Geometry: final body of the model. Coordinates: model frame, mm. Give positions to 0.01 mm unless a question says otherwise; leave off trailing zeros. Write each loop counter-clockwise with the first axis right and the second up, starting at its lowest first coordinate (ties: lowest second). Pieces come first, ordered by that corner, then holes. Notation, with made-up numbers: (-26, 79) -> (14, 79) arc R29 ccw to (14, 107) -> close; hole circle Ø6 at (-18.5, 13). An arc over 180 degrees is marked (long way). Answer in a Markdown table with one row per item. Add a question column.
Item 1: Section query B-B on x = -1.13. Output: boundary loops of the cut face in (y, z), plus the area to 3 significant figures.
Item 2: Section query D-D on y = 0.55. Output: boundary loops of the cut face in (x, z), plus the area to 3 significant figures.
Item 3: Section query A-A on z = -2. Output: boundary loops of the cut face in (x, y), plus the area to 3 significant figures.
Item 4: Material intervals for probe 1 along Z at (x, y) = (-0.65, 0.25); probe 2 along Y at (x, z) = (-1.45, 3.5); probe 3 along X at (y, z) = (-1.2, 3), sorted ascending. Write a range as from..to.
Item 5: First-contact query: P1, Ø2, axis at x = 1, z = 6.5, coming from the -Y side; P2, Ø2, axis at x = 1.5, z = -0.5, coming from the -Y side. Flat tips, straight axial feed; report the tip coordinate or a pass-through.
Item 6: Section query C-C on z = 2.5. Output: boundary loops of the cut face in (x, y).
```python
from build123d import *

# Parameters (mm, degrees)
SKETCH_1_R          = 2
EXTRUDE_1_DEPTH     = 8
SKETCH_2_R          = 0.2
EXTRUDE_2_DEPTH     = 3
SKETCH_3_W          = 0.679467602
SKETCH_3_H          = 0.176485091
CUT_EXTRUDE_1_DEPTH = 0.1
SKETCH_6_W          = 0.495308974
SKETCH_6_H          = 0.125078023
CUT_EXTRUDE_2_DEPTH = 0.1


with BuildPart() as part:
    # 草图1 → 凸台-拉伸1 (new body)
    with BuildSketch(Plane.XY):
        Circle(SKETCH_1_R)
    extrude(amount=EXTRUDE_1_DEPTH)

    # 草图2 → 凸台-拉伸2 (add)
    with BuildSketch(Plane(origin=(0, 0, 0), x_dir=(-1, 0, 0), z_dir=(0, 0, -1))):
        with Locations(Location((-1.13, 0, 0), (0, 0, 180))):
            Circle(SKETCH_2_R)
        with Locations(Location((1.13, 0, 0), (0, 0, 180))):
            Circle(SKETCH_2_R)
    extrude(amount=EXTRUDE_2_DEPTH)

    # 草图3 → 切除-拉伸1 (cut)
    with BuildSketch(Plane(origin=(2, 0, 0), x_dir=(0, 0, -1), z_dir=(1, 0, 0))):
        with Locations((-5.380383813, -0.002684697)):
            Rectangle(SKETCH_3_W, SKETCH_3_H)
        with Locations((-7.380383813, -0.002684697)):
            Rectangle(SKETCH_3_W, SKETCH_3_H)
        with Locations((-3.380383813, -0.002684697)):
            Rectangle(SKETCH_3_W, SKETCH_3_H)
        with Locations((-1.380383813, -0.002684697)):
            Rectangle(SKETCH_3_W, SKETCH_3_H)
    extrude(amount=-CUT_EXTRUDE_1_DEPTH, mode=Mode.SUBTRACT)

    # 草图6 → 切除-拉伸2 (cut)
    with BuildSketch(Plane.XY.offset(8)):
        with Locations((1.311678539, -0.002672358)):
            Rectangle(SKETCH_6_W, SKETCH_6_H)
        with Locations((0.311678539, -0.002672358)):
            Rectangle(SKETCH_6_W, SKETCH_6_H)
    extrude(amount=-CUT_EXTRUDE_2_DEPTH, mode=Mode.SUBTRACT)


solid = part.part
```
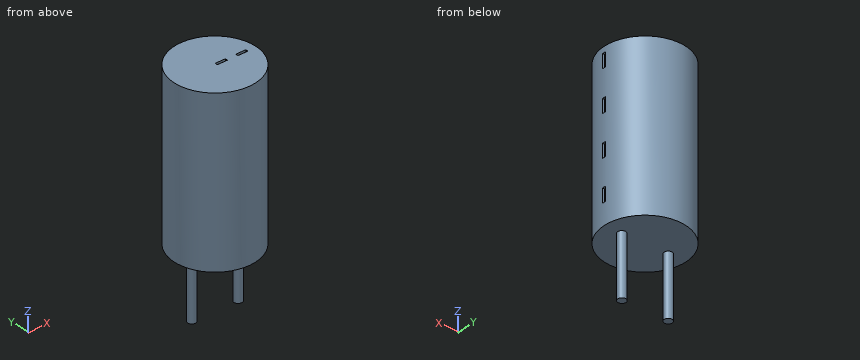
Findings below:
| question | item | result |
|---|---|---|
| 1 | outline | (-1.65, 0) -> (-0.2, 0) -> (-0.2, -3) -> (0.2, -3) -> (0.2, 0) -> (1.65, 0) -> (1.65, 8) -> (-1.65, 8) -> close |
| 1 | area | 27.6 mm^2 |
| 2 | outline | (-1.92, 0) -> (1.92, 0) -> (1.92, 8) -> (-1.92, 8) -> close |
| 2 | area | 30.8 mm^2 |
| 3 | outline | circle Ø0.4 at (-1.13, 0); circle Ø0.4 at (1.13, 0) |
| 3 | area | 0.251 mm^2 |
| 4 | probe 1 | z = 0..8 |
| 4 | probe 2 | y = -1.38..1.38 |
| 4 | probe 3 | x = -1.6..1.6 |
| 5 | P1 | stops at y = -2 |
| 5 | P2 | stops at y = -1.9 |
| 6 | outline | circle Ø4 at (0, 0) |
